CAD build for the part. Positions are in the model's coordinates, mm. A direction names the side the tool comes from. Coordinates: 2 decimals unless noted, no trailing zeros. Loops run counter-clockwise (first coordinate to the right, second up) from the corner with the lowest first, then second, coordinate; pieces in that order, holes last. Notation, with made-up numbers: (-11.75, 48.5) -> (36.25, 48.5) arc R28 ccw to (36.25, 83.5) -> close; hole circle Ø2 at (48.25, -3). An arc over 180 degrees is marked (long way). Write item = value, one per line. Start each with the question number.
(1) Drill centre lines: line 1 (Z direction, x = 0, y = -20.5); line 2 (X direction, y = -45, z = 0); line 3 (Z direction, x = 0, y = -0.8). Where is each one in solid material? Low to high. Write a range as from..to.
(2) Pull direction Z, two halves, no side cores. Call faces 3 (the face through (7, -50.8, 0)), 4 (the face through (-3.3, -37.28, -14.88)), 5 (the face through (1.93, -1.88, -8.68)): +Z half, -Z half, draft (parallel to the pull), parting line (faces both ways), or undercut.
(3) Band-saw the part on A-A (z = 0). Write the cut outline in (x, y).
(4) Flat gauge pins, fed straight in: P1, Ø4, axis at x = -2, z = -11.5, coming from the +Y side; P2, Ø8, axis at x = -8, y = -40.5, coming from the -Z side; P3, Ø4, axis at x = -4, y = -22.5, coming from the -Z side; P4, Ø10, axis at y = -12.5, z = 0, coming from the -X side. Where does each tip first touch, or does it go through?
(5) Band-saw the part on D-D (x = 11). Write the cut outline in (y, z).
(6) Tool access for faces 1 (the face through (-2, -3.81, -6)), 2 (the face through (5.718, -26.976, 1.801)): list every direction of +Z, -Z, +X, -X, +Y, -Y with a clear straight run to the whole face (end or side of a thin tool).
(7) Band-saw the part on C-C (y = -41.5). Write the cut outline in (x, z), and give its area (3 significant figures).
(8) Band-saw the part on B-B (x = 0). Write the cut outline in (y, z), and give its area (3 significant figures).
```python
from build123d import *

# Parameters (mm, degrees)
F0_R     = 15.24
F0_R_2   = 5.9944
F1_DEPTH = 50.8
F2_R     = 18.435252
F2_R_2   = 12.7
F3_DEPTH = 24.13
F4_R     = 8.89
F5_DEPTH = 3.81


with BuildPart() as f1:
    # F0 (on Front) → F1 (new body)
    with BuildSketch(Plane.XZ):
        Circle(F0_R)
        Circle(F0_R_2, mode=Mode.SUBTRACT)
    extrude(amount=F1_DEPTH)

    # F2 (on face) → F3 (cut)
    with BuildSketch(Plane(origin=(0, 0, 0), x_dir=(-1, 0, 0), z_dir=(0, 1, 0))):
        Circle(F2_R)
        Circle(F2_R_2, mode=Mode.SUBTRACT)
    extrude(amount=-F3_DEPTH, mode=Mode.SUBTRACT)

    # F4 (on face) → F5 (cut)
    with BuildSketch(Plane(origin=(0, 0, 0), x_dir=(-1, 0, 0), z_dir=(0, 1, 0))):
        Circle(F4_R)
    extrude(amount=-F5_DEPTH, mode=Mode.SUBTRACT)


solid = f1.part
```
Findings below:
q1.line_1 = -12.7..-5.99, 5.99..12.7
q1.line_2 = -15.24..-5.99, 5.99..15.24
q1.line_3 = -12.7..-8.89, 8.89..12.7
q2.face_3 = draft
q2.face_4 = parting line
q2.face_5 = undercut
q3.outline = (-15.24, -50.8) -> (-5.99, -50.8) -> (-5.99, -3.81) -> (-8.89, -3.81) -> (-8.89, 0) -> (-12.7, 0) -> (-12.7, -24.13) -> (-15.24, -24.13) -> close; (5.99, -50.8) -> (15.24, -50.8) -> (15.24, -24.13) -> (12.7, -24.13) -> (12.7, 0) -> (8.89, 0) -> (8.89, -3.81) -> (5.99, -3.81) -> close
q4.P1 = 0
q4.P2 = -14.71
q4.P3 = -14.97
q4.P4 = -12.7
q5.outline = (-50.8, -10.55) -> (-24.13, -10.55) -> (-24.13, -6.35) -> (0, -6.35) -> (0, 6.35) -> (-24.13, 6.35) -> (-24.13, 10.55) -> (-50.8, 10.55) -> close
q6.face_1 = +Y
q6.face_2 = +Y, -Y
q7.outline = circle Ø30.48 at (0, 0); hole circle Ø11.99 at (0, 0)
q7.area = 617 mm²
q8.outline = (-50.8, -15.24) -> (-24.13, -15.24) -> (-24.13, -12.7) -> (0, -12.7) -> (0, -8.89) -> (-3.81, -8.89) -> (-3.81, -5.99) -> (-50.8, -5.99) -> close; (-50.8, 5.99) -> (-3.81, 5.99) -> (-3.81, 8.89) -> (0, 8.89) -> (0, 12.7) -> (-24.13, 12.7) -> (-24.13, 15.24) -> (-50.8, 15.24) -> close
q8.area = 795 mm²
